```python
from build123d import *

# Parameters (mm, degrees)
F0_R     = 70.868501
F1_DEPTH = 6.35
F2_DEPTH = 10.16
F3_DEPTH = 12.7


with BuildPart() as f1:
    # F0 (on Top) → F1 (new body)
    with BuildSketch(Plane.XY):
        Circle(F0_R)
        Polygon((-27.191779, -33.847008), (-27.535122, 34.270629), (-22.413259, 34.270629), (-22.014963, -33.816725), align=None, mode=Mode.SUBTRACT)
        Polygon((-11.780724, 3.469003), (7.036994, 3.577667), (7.036994, -1.531884), (-11.780724, -1.798139), align=None, mode=Mode.SUBTRACT)
        Polygon((10.873231, -17.685675), (31.554632, 31.392667), (36.254622, 29.430676), (15.738306, -19.71658), align=None, mode=Mode.SUBTRACT)
    extrude(amount=F1_DEPTH)

    # F0 (on Top) → F2 (join)
    with BuildSketch(Plane.XY):
        Polygon((-22.413259, 34.270629), (-27.535122, 34.270629), (-27.191779, -33.847008), (-22.014963, -33.816725), align=None)
        Polygon((7.036994, -1.531884), (7.036994, 3.577667), (-11.780724, 3.469003), (-11.780724, -1.798139), align=None)
    extrude(amount=F2_DEPTH)

    # F0 (on Top) → F3 (join)
    with BuildSketch(Plane.XY):
        Polygon((36.254622, 29.430676), (31.554632, 31.392667), (10.873231, -17.685675), (15.738306, -19.71658), align=None)
    extrude(amount=F3_DEPTH)


solid = f1.part
```
The listing builds one solid part. Answer for the finished solid, in the listing's coordinates (mm). A direction names the side the tool comes from. Round coordinates to 2 decimals unless told otherwise and drop trailing zeros. Write each loop counter-clockwise with the first axis right and the second up, starting at its lowest first coordinate (ties: lowest second). Pieces come first, ordered by that corner, then holes. Notation, with made-up numbers: (11.25, -21.75) -> (68.25, -21.75) arc R17 cw to (68.25, -14.75) -> close; hole circle Ø4 at (38, 54). An arc over 180 degrees is marked (long way). Use CSV: the item, a comma, the result in double quotes. Start each with the question number.
(1) Which of the six approach directions +Z, -Z, +X, -X, +Y, -Y give full straight-line access (tool end or side, diameter ignored) to faces 5 (the face through (21.36, 7.2, 9.48)), 6 (the face through (25.85, 4.51, 9.48)), 7 (the face through (-3, 1, 10.16)), 8 (the face through (7.037, 1, 8)), 9 (the face through (-25, 34.271, 8))?
(2) Section D-D on y = -30 is taken. Give the vertices of the cut face in (x, z).
(3) Section A-A on z = 8.25 is taken. Give the vertices of the cut face in (x, y).
(4) The mould has two halves that part along X. Classify faces 1 (the face through (13.3, -18.7, 9.5)), 2 (the face through (24, 6, 12.7)), 3 (the face through (33.938, 30.398, 9.481)), 4 (the face through (67.596, 21.287, 3.131)): released by +X, released by -X, zero draft, split by the parting line, or undercut.
(5) Each of these flat-tipped pins is pushed along its axis until it touches: pin 1 (4.5 mm diameter, centred on x = -25, y = 1, fed in from +Z); pin 2 (1 mm diameter, centred on y = -39, z = 3.5, fed in from +X); pin 3 (5 mm diameter, centred on y = -18, z = 4.5, fed in from -X). Where does it stop, or does it pass through?
(6) Section C-C on x = 0 is taken. Give the vertices of the cut face in (y, z).
(7) Section B-B on y = 8 is taken. Give the vertices of the cut face in (x, z).
(8) Consider L1, parallel to Z at x = -7, y = 35.5; L2, parallel to Z at x = -23, y = -25; L3, parallel to X at y = 3, z = 8. Determine where each line is inside the solid, lowest interval first. Write a range as from..to.
A:
1,face 5,"+Z, +Y"
1,face 6,"+Z, +X, -Y"
1,face 7,"+Z, -X, +Y, -Y"
1,face 8,"+Z, +Y, -Y"
1,face 9,"+Z, +X, -X, +Y"
2,outline,"(-64.21, 0) -> (64.21, 0) -> (64.21, 6.35) -> (-22.04, 6.35) -> (-22.04, 10.16) -> (-27.21, 10.16) -> (-27.21, 6.35) -> (-64.21, 6.35) -> close"
3,outline,"(-27.54, 34.27) -> (-27.19, -33.85) -> (-22.01, -33.82) -> (-22.41, 34.27) -> close; (-11.78, -1.8) -> (7.04, -1.53) -> (7.04, 3.58) -> (-11.78, 3.47) -> close; (10.87, -17.69) -> (15.74, -19.72) -> (36.25, 29.43) -> (31.55, 31.39) -> close"
4,face 1,"undercut"
4,face 2,"zero draft"
4,face 3,"released by +X"
4,face 4,"split by the parting line"
5,pin 1,"stops at z = 10.16"
5,pin 2,"stops at x = 59.5"
5,pin 3,"stops at x = -69.15"
6,outline,"(-70.87, 0) -> (70.87, 0) -> (70.87, 6.35) -> (3.54, 6.35) -> (3.54, 10.16) -> (-1.63, 10.16) -> (-1.63, 6.35) -> (-70.87, 6.35) -> close"
7,outline,"(-70.42, 0) -> (70.42, 0) -> (70.42, 6.35) -> (27.31, 6.35) -> (27.31, 12.7) -> (21.7, 12.7) -> (21.7, 6.35) -> (-22.26, 6.35) -> (-22.26, 10.16) -> (-27.4, 10.16) -> (-27.4, 6.35) -> (-70.42, 6.35) -> close"
8,L1,"z = 0..6.35"
8,L2,"z = 0..10.16"
8,L3,"x = -27.38..-22.23, -11.78..7.04, 19.59..25.22"
